For this review, take the finished solid that the model builds, in its own axes (mm). Face numbers are marked on the shaded views. A direction names the side the tool comes from. Coordinates: 2 decimals unless noted, no trailing zeros. Order: outer loops, then holes, each group sorted by start corner. A loop starts at its lowest first (then second) coordinate and runs counter-clockwise, first axis right, second up. Notation, with made-up numbers: (77.5, 1) -> (102.5, 1) arc R28 ccw to (102.5, 27) -> close; hole circle Ø6 at (-28, 44.5). An arc over 180 degrees is marked (long way). Answer as a JSON object with one key per item and string values. Group by question number.
1) Wall thickness on L1, parallel to X at y = 20.5, z = 24.5 (3 decimals); L2, parallel to Y at x = 69, z = 21; L3, parallel to Y at x = 101, z = 24: over which ranges is each line inside the solid? List them lowest first.
2) Add section C-C, the plane y = 29. Write out the cut boundary in (x, z) (3 decimals), then the cut area to 3 significant figures.
3) For pin 1 (5 mm diameter, centred on y = 128, z = 21, fed in from +X); pin 2 (3.5 mm diameter, centred on x = 134.5, z = 13, fed in from +Y); pin 3 (2 mm diameter, centred on x = 105.5, z = 8, fed in from +Y), all flat-tipped, find the tip position at first contact; note any pin that passes through.
4) Add section D-D, the plane x = 69.85. Write out the cut boundary in (y, z), then the cut area to 3 significant figures.
5) Add section A-A, the plane x = 94.5. Write out the cut boundary in (y, z), then the cut area to 3 significant figures.
6) Draft analysis for pull direction Y (two halves, no side actions). For the marked faces 1, 2 and 3, state which applies: +Y half, -Y half, draft (parallel to the pull), parting line (faces both ways), or undercut.
7) Machinability: for the marked faces 4, 5, 6 and 7, which of the approach directions +Z, -Z, +X, -X, +Y, -Y give a long, thin tool a straight path to every point of the face, cutting with its end or side? Answer none if there is none.
from build123d import *

# Parameters (mm, degrees)
F1_DEPTH = 38.1


with BuildPart() as f1:
    # F0 (on Top) → F1 (new body)
    with BuildSketch(Plane.XY):
        with BuildLine():
            ThreePointArc((0, 1.5875), (0.464968, 0.464968), (1.5875, 0))
            Line((1.5875, 0), (138.1125, 0))
            ThreePointArc((138.1125, 0), (139.235032, 0.464968), (139.7, 1.5875))
            Line((139.7, 1.5875), (139.7, 11.1125))
            ThreePointArc((139.7, 11.1125), (139.235032, 12.235032), (138.1125, 12.7))
            Line((138.1125, 12.7), (127, 12.7))
            ThreePointArc((127, 12.7), (124.754936, 13.629936), (123.825, 15.875))
            Line((123.825, 15.875), (123.825, 66.802))
            ThreePointArc((123.825, 66.802), (115.346997, 95.842039), (92.576316, 115.759279))
            ThreePointArc((92.576316, 115.759279), (89.897412, 118.102484), (88.9, 121.518959))
            Line((88.9, 121.518959), (88.9, 131.7625))
            ThreePointArc((88.9, 131.7625), (88.435032, 132.885032), (87.3125, 133.35))
            Line((87.3125, 133.35), (77.7875, 133.35))
            ThreePointArc((77.7875, 133.35), (76.664968, 132.885032), (76.2, 131.7625))
            Line((76.2, 131.7625), (76.2, 109.052363))
            ThreePointArc((76.2, 109.052363), (76.565724, 108.038746), (77.494387, 107.492158))
            ThreePointArc((77.494387, 107.492158), (69.85, 25.4), (62.205613, 107.492158))
            ThreePointArc((62.205613, 107.492158), (63.134276, 108.038746), (63.5, 109.052363))
            Line((63.5, 109.052363), (63.5, 131.7625))
            ThreePointArc((63.5, 131.7625), (63.035032, 132.885032), (61.9125, 133.35))
            Line((61.9125, 133.35), (52.3875, 133.35))
            ThreePointArc((52.3875, 133.35), (51.264968, 132.885032), (50.8, 131.7625))
            Line((50.8, 131.7625), (50.8, 121.518959))
            ThreePointArc((50.8, 121.518959), (49.802588, 118.102484), (47.123684, 115.759279))
            ThreePointArc((47.123684, 115.759279), (24.353003, 95.842039), (15.875, 66.802))
            Line((15.875, 66.802), (15.875, 15.875))
            ThreePointArc((15.875, 15.875), (14.945064, 13.629936), (12.7, 12.7))
            Line((12.7, 12.7), (1.5875, 12.7))
            ThreePointArc((1.5875, 12.7), (0.464968, 12.235032), (0, 11.1125))
            Line((0, 11.1125), (0, 1.5875))
        make_face()
    extrude(amount=F1_DEPTH)


solid = f1.part
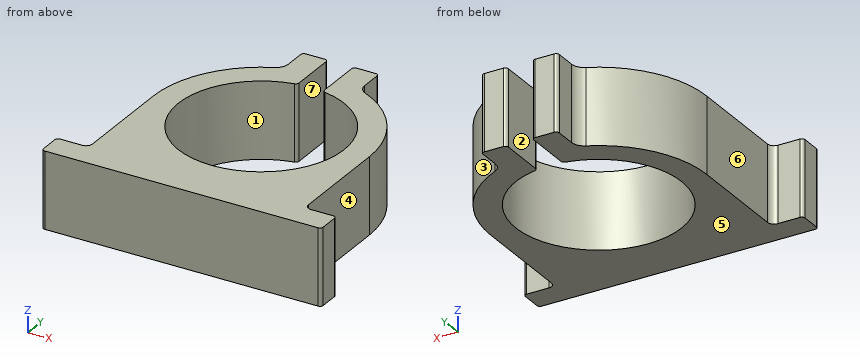
Output values:
{
 "1": {"L1": "x = 15.875 to 123.825", "L2": "y = 0 to 25.41", "L3": "y = 0 to 39.53, 94.07 to 110.88"},
 "2": {"outline": "(15.875, 0) -> (52.964, 0) -> (52.964, 38.1) -> (15.875, 38.1) -> close; (86.736, 0) -> (123.825, 0) -> (123.825, 38.1) -> (86.736, 38.1) -> close", "area": "2,830 mm²"},
 "3": {"pin 1": "stops at x = 88.9", "pin 2": "stops at y = 12.7", "pin 3": "stops at y = 108.19"},
 "4": {"outline": "(0, 0) -> (25.4, 0) -> (25.4, 38.1) -> (0, 38.1) -> close", "area": "968 mm²"},
 "5": {"outline": "(0, 0) -> (33.54, 0) -> (33.54, 38.1) -> (0, 38.1) -> close; (100.07, 0) -> (114.82, 0) -> (114.82, 38.1) -> (100.07, 38.1) -> close", "area": "1,840 mm²"},
 "6": {"face 1": "undercut", "face 2": "draft", "face 3": "+Y half"},
 "7": {"face 4": "+Z, -Z, +X, +Y", "face 5": "-Z, +X, -X, +Y, -Y", "face 6": "+Z, -Z, -X, +Y", "face 7": "+Z, -Z, +Y"}
}
